Here's how the part is built. I have some questions about the finished solid (model axes, mm). A direction names the side the tool comes from. Round coordinates to 2 decimals unless told otherwise and drop trailing zeros. Write each loop counter-clockwise with the first axis right and the second up, starting at its lowest first coordinate (ties: lowest second). Pieces come first, ordered by that corner, then holes. Notation, with made-up numbers: (60, -29.5) - (100, -29.5) arc R14 ccw to (100, -21.5) - close; hole circle Ø10 at (54.25, 46). An arc over 180 degrees is marked (long way). Return JSON: item names as keys, results as strings. Group by question number.
```python
from build123d import *

# Parameters (mm, degrees)
F1_DEPTH = 2.5


with BuildPart() as f1:
    # F0 (on Top) → F1 (new body)
    with BuildSketch(Plane.XY):
        with BuildLine():
            Line((-22, 58.75), (0, 58.75))
            Line((0, 58.75), (0, 65.75))
            Line((0, 65.75), (-23.68421, 65.75))
            ThreePointArc((-23.68421, 65.75), (-26.735934, 64.485934), (-28, 61.43421))
            Line((-28, 61.43421), (-28, -61.43421))
            ThreePointArc((-28, -61.43421), (-26.735934, -64.485934), (-23.68421, -65.75))
            Line((-23.68421, -65.75), (0, -65.75))
            Line((0, -65.75), (0, -58.75))
            Line((0, -58.75), (-22, -58.75))
            Line((-22, -58.75), (-22, -13.75))
            Line((-22, -13.75), (-26.5, -13.75))
            Line((-26.5, -13.75), (-26.5, 13.75))
            Line((-26.5, 13.75), (-22, 13.75))
            Line((-22, 13.75), (-22, 58.75))
        make_face()
    extrude(amount=F1_DEPTH)


solid = f1.part
```
1) Will these pins go through, and if not, where does the flat tip stop? pin 1 Ø0.8 at (y, z) = (-26.5, 1.5) entering from +X; pin 2 Ø1.2 at (x, z) = (-25, 1) entering from +Y; pin 3 Ø0.8 at (y, z) = (0, 1) entering from +X.
2) For faces 1 (the flat face through (-24, 13.75, 1)), 2 (the flat face through (-12, 65.75, 1)), which set-ups out of +Z, -Z, +X, -X, +Y, -Y let a thin tool reach every point of the face, with its end or its side?
3) Imagine slicing it at B-B (z = 1.1). Please give me the cut outline in (x, y).
4) Imagine slicing it at A-A (x = -19.75). Please give me the cut outline in (y, z).
5) Imagine slicing it at C-C (y = -4). Please give me the cut outline in (x, z).
6) Imagine slicing it at D-D (y = 26.5). Please give me the cut outline in (x, z), plus the area to 3 significant figures.
7) If we mould it in two halves opening along Y, with no side actions, what happens to faces 3 (the flat face through (-22, 36, 1)), 4 (the cylindrical face through (-26.7, 64.52, 1.23)), 5 (the flat face through (-28, 1, 1))? For each: released by +Y, released by -Y, zero draft, split by the parting line, or undercut.
8) I need wall thicknesses on line 1 along Y through (x, z) = (-17.25, 2.25); line 2 along X through (y, z) = (22, 2.2); line 3 along Y through (x, z) = (-24.75, 1.55). Which ranges of each line are inside material? Lowest first, please.
Results found:
{
 "1": {"pin 1": "stops at x = -22", "pin 2": "stops at y = 65.69", "pin 3": "stops at x = -26.5"},
 "2": {"face 1": "+Z, -Z, +X", "face 2": "+Z, -Z, +X, -X, +Y"},
 "3": {"outline": "(-28, -61.43) arc R4.32 ccw to (-23.68, -65.75) - (0, -65.75) - (0, -58.75) - (-22, -58.75) - (-22, -13.75) - (-26.5, -13.75) - (-26.5, 13.75) - (-22, 13.75) - (-22, 58.75) - (0, 58.75) - (0, 65.75) - (-23.68, 65.75) arc R4.32 ccw to (-28, 61.43) - close"},
 "4": {"outline": "(-65.75, 0) - (-58.75, 0) - (-58.75, 2.5) - (-65.75, 2.5) - close; (58.75, 0) - (65.75, 0) - (65.75, 2.5) - (58.75, 2.5) - close"},
 "5": {"outline": "(-28, 0) - (-26.5, 0) - (-26.5, 2.5) - (-28, 2.5) - close"},
 "6": {"outline": "(-28, 0) - (-22, 0) - (-22, 2.5) - (-28, 2.5) - close", "area": "15.0 mm²"},
 "7": {"face 3": "undercut", "face 4": "released by +Y", "face 5": "zero draft"},
 "8": {"line 1": "y = -65.75 to -58.75, 58.75 to 65.75", "line 2": "x = -28 to -22", "line 3": "y = -65.62 to -13.75, 13.75 to 65.62"}
}
